Can you work these out from the model? Positions are in its coordinate system, mm. A direction names the side the tool comes from. Give positions to 0.01 mm unless a question says otherwise; leave off trailing zeros. Order: outer loops, then holes, each group sorted by start corner. A loop starts at its lowest first (then second) coordinate and runs counter-clockwise, first axis right, second up. Notation, with made-up numbers: (-10, -16) -> (10, -16) arc R20 cw to (10, 20) -> close; hole circle Ø7 at (77, -3.75). An arc over 180 degrees is marked (long way). Answer as a JSON object with one key per item and string values.
Autodesk Inventor part; units mm, degrees
ref_plane "YZ Plane" through (0, 0, 0) normal (1, 0, 0) x (0, 1, 0)
ref_plane "XZ Plane" through (0, 0, 0) normal (0, 1, 0) x (-1, 0, 0)
ref_plane "XY Plane" through (0, 0, 0) normal (0, 0, 1) x (1, 0, 0)
sketch "Skizze1" plane through (0, 0, 0) normal (1, 0, 0) x (0, 1, 0)
  line L0 (0, 0) -> (0, -45)
  line L1 (0, -45) -> (65, -45)
  line L2 (65, -45) -> (65, -42.5)
  line L3 (65, -42.5) -> (2.5, -42.5)
  line L4 (2.5, -42.5) -> (2.5, 0)
  line L5 (2.5, 0) -> (0, 0)
  dimension "d0" = 45
  dimension "d1" = 65
  dimension "d2" = 2.5
  dimension "d3" = 62.5
extrude "Extrusion1" add sketch "Skizze1" along normal mid plane 60
sketch "Skizze2" plane through (-30, 2.5, 0) normal (0, 1, 0) x (1, 0, 0)
  circle A0 centre (7.5, 21.25) radius 2.75
  circle A1 centre (52.5, 22.5) radius 2.75
  point P0 (30, 0)
  dimension "d6" = 5.5
  dimension "d7" = 5.5
extrude "Extrusion2" cut sketch "Skizze2" against normal blind 3
sketch "Skizze3" plane through (-30, 2.5, -42.5) normal (0, 0, 1) x (1, 0, 0)
  circle A0 centre (30, 32.2) radius 19.075
  circle A1 centre (56.25, 58.75) radius 2.25
  line L0 (0, 62.5) -> (60, 62.5)
  circle A2 centre (3.75, 3.75) radius 2.25
  circle A3 centre (56.25, 3.75) radius 2.25
  circle A4 centre (3.75, 58.45) radius 2.25
  point P0 (30, -2.5)
  dimension "d10" = 38.15
  dimension "d11" = 4.5
  dimension "d12" = 3.75
  dimension "d13" = 4.5
  dimension "d14" = 4.5
  dimension "d15" = 4.5
extrude "Extrusion3" cut sketch "Skizze3" against normal blind 2.5
properties part number "Motorhalterung"
1. If we section it at B-B on y = 34.7: Please give me the cut outline in (x, z) (3 decimals), then the cut area to 3 significant figures.
Worked answers:
{"outline": "(-30, -45) -> (-19.075, -45) -> (-19.075, -42.5) -> (-30, -42.5) -> close; (19.075, -45) -> (30, -45) -> (30, -42.5) -> (19.075, -42.5) -> close", "area": "54.6 mm²"}
2. For faces 4 (the face through (27.288, 59.254, -43.732)), 5 (the face through (0, 2.5, -22)), which set-ups out of +Z, -Z, +X, -X, +Y, -Y let a thin tool reach every point of the face, with its end or its side?
Worked answers:
{"face 4": "+Z, -Z", "face 5": "+Z, +X, -X, +Y"}
3. If we section it at A-A on x = -22.5: Please give me the cut outline in (y, z).
Worked answers:
{"outline": "(0, -45) -> (65, -45) -> (65, -42.5) -> (2.5, -42.5) -> (2.5, -24) -> (0, -24) -> close; (0, -18.5) -> (2.5, -18.5) -> (2.5, 0) -> (0, 0) -> close"}
4. If we section it at C-C on z = -22.5: Please give me the cut outline in (x, y), then the cut area to 3 significant figures.
Worked answers:
{"outline": "(-30, 0) -> (-24.95, 0) -> (-24.95, 2.5) -> (-30, 2.5) -> close; (-20.05, 0) -> (19.75, 0) -> (19.75, 2.5) -> (-20.05, 2.5) -> close; (25.25, 0) -> (30, 0) -> (30, 2.5) -> (25.25, 2.5) -> close", "area": "124 mm²"}
5. Will these pins go through, and if not, where does the flat tip stop? pin 1 Ø3 at (x, z) = (-23, -18.5) entering from -Y; pin 2 Ø3.5 at (x, z) = (22.5, -22.5) entering from -Y; pin 3 Ø2 at (x, y) = (-12.5, 51) entering from +Z; pin 4 Ø2 at (x, z) = (-22.5, -14) entering from +Y.
Worked answers:
{"pin 1": "y = 0", "pin 2": "through", "pin 3": "z = -42.5", "pin 4": "y = 2.5"}
6. Please list where these lines run through material, in increasing order: L1, parallel to Y at x = 26, z = -43; L2, parallel to Z at x = -22.5, y = 0.9; L3, parallel to Y at x = -26.25, z = -43.7.
Worked answers:
{"L1": "0 to 4.01, 8.49 to 59.01, 63.49 to 65", "L2": "-45 to -24, -18.5 to 0", "L3": "0 to 4, 8.5 to 58.7, 63.2 to 65"}
7. If we mould it in two halves opening along Y, with no side actions, what happens to faces 1 (the face through (19.753, 1.268, -22.621)), 2 (the face through (28.396, 6.926, -43.732)), 3 (the face through (0, 65, -44))? For each: +Y half, -Y half, draft (parallel to the pull), parting line (faces both ways), or undercut.
Worked answers:
{"face 1": "draft", "face 2": "undercut", "face 3": "+Y half"}
8. If we section it at D-D on y = 6.25: Please give me the cut outline in (x, z), then the cut area to 4 significant figures.
Worked answers:
{"outline": "(-30, -45) -> (-28.5, -45) -> (-28.5, -42.5) -> (-30, -42.5) -> close; (-24, -45) -> (24, -45) -> (24, -42.5) -> (-24, -42.5) -> close; (28.5, -45) -> (30, -45) -> (30, -42.5) -> (28.5, -42.5) -> close", "area": "127.5 mm²"}
